The drawing under review shows one solid part. Ordinate dimensions are in mm from its lowest x, y, z. Give positions to 0.01 mm unless a question says otherwise; leave off trailing zeros. Order: outer loops, then holes, each group sorted by start corner. A loop starts at its lowest first (then second) coordinate and runs counter-clockwise, first axis right, second up. Notation, with made-up numbers: (10.25, -23.75) -> (62.25, -23.75) arc R14 cw to (62.25, 3.25) -> close; hole circle Ø8 at (11, -9.75). An arc over 180 degrees is marked (long way). One line per item, written item: value. Start each with the question number.
1) Consider section B-B (y = 25.5). State the section outline as (x, z) points.
2) Consider section C-C (z = 1.9). State the section outline as (x, y) points, plus the area to 3 significant figures.
3) Wall thickness on line 1 along X through (y, z) = (32.5, 3); line 2 along X through (y, z) = (14, 2.5); line 3 along Y through (x, z) = (14, 2.85): over which ranges is each line inside the solid? List them lowest first. Write a range as from..to.
4) For pin 1 (4 mm diameter, centred on x = 13, y = 28, fed in from -Z); pin 2 (1.5 mm diameter, centred on x = 3.5, z = 3.5, fed in from +Y); pin 3 (1.5 mm diameter, centred on x = 51.5, z = 3.5, fed in from +Y); pin 4 (1.5 mm diameter, centred on x = 25, z = 3, fed in from -Y), all flat-tipped, find the tip position at first contact; note any pin that passes through.
5) Consider section A-A (y = 4). State the section outline as (x, z) points, plus the area to 3 significant figures.
6) Consider section D-D (x = 100.5). State the section outline as (y, z) points.
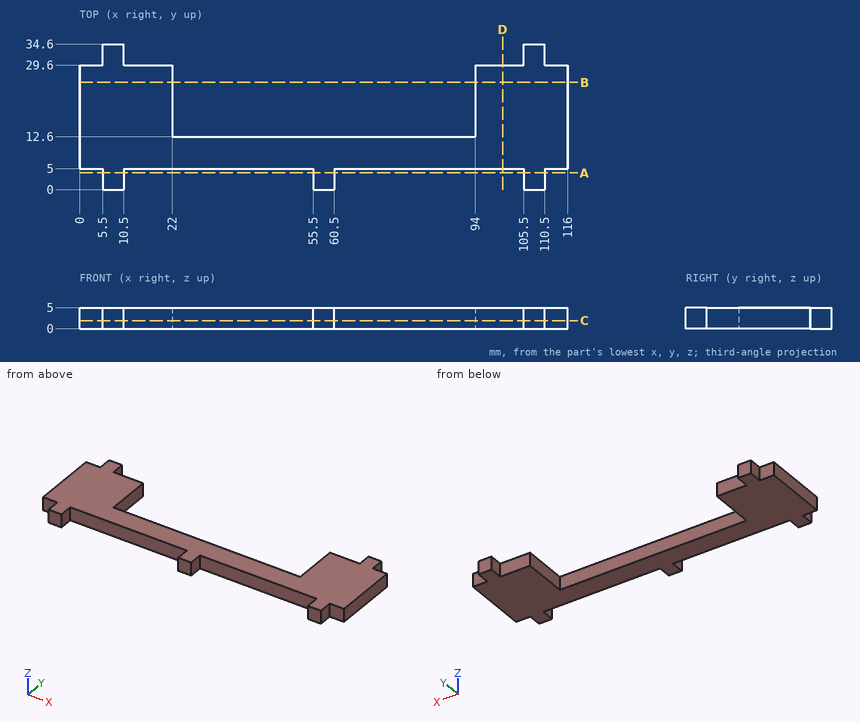
Checked values:
1. outline: (0, 0) -> (22, 0) -> (22, 5) -> (0, 5) -> close; (94, 0) -> (116, 0) -> (116, 5) -> (94, 5) -> close
2. outline: (0, 5) -> (5.5, 5) -> (5.5, 0) -> (10.5, 0) -> (10.5, 5) -> (55.5, 5) -> (55.5, 0) -> (60.5, 0) -> (60.5, 5) -> (105.5, 5) -> (105.5, 0) -> (110.5, 0) -> (110.5, 5) -> (116, 5) -> (116, 29.6) -> (110.5, 29.6) -> (110.5, 34.6) -> (105.5, 34.6) -> (105.5, 29.6) -> (94, 29.6) -> (94, 12.6) -> (22, 12.6) -> (22, 29.6) -> (10.5, 29.6) -> (10.5, 34.6) -> (5.5, 34.6) -> (5.5, 29.6) -> (0, 29.6) -> close
2. area: 1,750 mm^2
3. line 1: x = 5.5..10.5, 105.5..110.5
3. line 2: x = 0..22, 94..116
3. line 3: y = 5..29.6
4. pin 1: stops at z = 0
4. pin 2: stops at y = 29.6
4. pin 3: stops at y = 12.6
4. pin 4: stops at y = 5
5. outline: (5.5, 0) -> (10.5, 0) -> (10.5, 5) -> (5.5, 5) -> close; (55.5, 0) -> (60.5, 0) -> (60.5, 5) -> (55.5, 5) -> close; (105.5, 0) -> (110.5, 0) -> (110.5, 5) -> (105.5, 5) -> close
5. area: 75.0 mm^2
6. outline: (5, 0) -> (29.6, 0) -> (29.6, 5) -> (5, 5) -> close
